Verification items for the finished model (mm, model axes). Round coordinates to 2 decimals unless told otherwise and drop trailing zeros.
Autodesk Inventor part; units mm, degrees
ref_plane "YZ Plane" through (0, 0, 0) normal (1, 0, 0) x (0, 1, 0)
ref_plane "XZ Plane" through (0, 0, 0) normal (0, 1, 0) x (-1, 0, 0)
ref_plane "XY Plane" through (0, 0, 0) normal (0, 0, 1) x (1, 0, 0)
sketch "Sketch1" plane through (0, 0, 0) normal (0, 0, 1) x (1, 0, 0)
  line L0 (0, 217.805) -> (0, -217.805)
  line L1 (-302.26, 0) -> (302.26, 0)
  line L2 (215.9, -155.575) -> (-215.9, -155.575)
  line L3 (-215.9, -155.575) -> (-215.9, 155.575)
  line L4 (-215.9, 155.575) -> (215.9, 155.575)
  line L5 (215.9, 155.575) -> (215.9, -155.575)
  line L6 (215.9, -155.575) -> (-215.9, 155.575) construction
  line L7 (-215.9, -155.575) -> (215.9, 155.575) construction
  line L8 (186.69, -13.13) -> (186.69, -35.13) construction
  line L9 (189.23, 88.9) -> (189.23, 63.5) construction
  line L10 (189.23, -63.5) -> (189.23, -88.9) construction
  point P0 (0, 0)
  point P1 (-203.2, 123.818)
  point P2 (-203.2, 95.818)
  point P3 (-203.2, -108.525)
  point P4 (-203.2, -136.525)
  point P5 (165.1, 46.8376)
  point P6 (165.1, -46.8376)
  point P7 (186.69, -24.13)
  point P8 (189.23, -76.2)
  point P9 (189.23, 76.2)
  dimension "d0" = 311.15
  dimension "d1" = 431.8
  dimension "d2" = 28
  dimension "d3" = 28
  dimension "d4" = 203.2
  dimension "d16" = 204.343
  dimension "d17" = 19.05
  dimension "d18" = 31.757
  dimension "d19" = 93.6752
  dimension "d20" = 46.8376
  dimension "d21" = 165.1
  dimension "d29" = 22
  dimension "d31" = 186.69
  dimension "d44" = 25.4
  dimension "d45" = 25.4
  dimension "d46" = 24.13
  dimension "d47" = 76.2
  dimension "d48" = 76.2
  dimension "d57" = 189.23
extrude "Extrusion1" add sketch "Sketch1" against normal blind 6.35
hole "Hole1-Tap M5" at (-203.2, 123.818, 0) at (-203.2, 95.818, 0) at (-203.2, -108.525, 0) at (-203.2, -136.525, 0) direction (0, 0, -1) diameter 4.064 end through all
hole "Hole2-Tap M5" at (165.1, 46.8376, 0) at (165.1, -46.8376, 0) direction (0, 0, -1) diameter 4.064 end through all
hole "Hole3-Tap M4" at (186.69, -13.13, 0) at (186.69, -35.13, 0) direction (0, 0, -1) diameter 3.1242 end through all
fillet "Fillet1" radius 9.525 4 edges at (-215.9, 155.575, -3.175) (215.9, 155.575, -3.175) (215.9, -155.575, -3.175) (-215.9, -155.575, -3.175)
hole "Hole4 CSINK M4" at (189.23, -88.9, 0) at (189.23, 88.9, 0) at (189.23, 63.5, 0) at (189.23, -63.5, 0) direction (0, 0, -1) diameter 4.4958 end through all countersink diameter 9.398 countersink angle 90
properties material "ACRYLIC, CLEAR"
1. Gauge pin test, flat ends, axial feed: P1, Ø1.9, axis at x = 186.69, y = -35.13, coming from the -Z side; P2, Ø5, axis at x = 189.23, y = -88.9, coming from the +Z side. Record the tip position at first contact, or that the pin passes through.
2. Release check for a two-part mould opening along Y. For faces 1 (the face through (190.85, 90.67, -2.3)), 2 (the face through (189.95, -65.79, -2.3)), 3 (the face through (-213.036, -152.859, -3.219)), 4 (the face through (213.036, 152.859, -3.219)) record: released by +Y, released by -Y, zero draft, split by the parting line, or undercut.
3. Scan lines: L1, parallel to Y at x = -203.2, z = -5 (3 decimals); L2, parallel to Y at x = 165.1, z = -2.25 (3 decimals); L3, parallel to X at y = -88.9, z = -4.15. Record each from-to range of solid material in increasing order.
Taken from the geometry:
1. P1: passes through
1. P2: stops at z = -2.2
2. face 1: undercut
2. face 2: undercut
2. face 3: released by -Y
2. face 4: released by +Y
3. L1: y = -155.575 to -138.557, -134.493 to -110.557, -106.493 to 93.786, 97.85 to 121.786, 125.85 to 155.575
3. L2: y = -155.575 to -48.87, -44.806 to 44.806, 48.87 to 155.575
3. L3: x = -215.9 to 186.98, 191.48 to 215.9
